```python
from build123d import *

# Parameters (mm, degrees)
SKETCH1_W                  = 812.8
SKETCH1_H                  = 77.724
BOSS_EXTRUDE1_DEPTH        = 22.225
SKETCH2_W                  = 71.374
SKETCH2_H                  = 19.05
CUT_EXTRUDE1_DEPTH         = 817.364663535
HOLE1_D                    = 9.652
HOLE2_D                    = 28.575
H_0_266_DIAMETER_HOLE1_D   = 6.7564
F_10_CLEARANCE_HOLE1_D     = 5.334
F_10_CLEARANCE_HOLE1_DEPTH = 3.175
F_10_CLEARANCE_HOLE2_D     = 5.334
F_10_CLEARANCE_HOLE2_DEPTH = 3.175
F_10_CLEARANCE_HOLE3_D     = 5.334
CHAMFER1_SIZE              = 3.175
FILLET1_R                  = 0.762
FILLET2_R                  = 3.937
CUT_EXTRUDE2_REACH         = 818.445
SKETCH15_W                 = 23.8125
SKETCH15_H                 = 77.724


with BuildPart() as part:
    # Sketch1 → Boss-Extrude1 (new body)
    with BuildSketch(Plane.XZ.offset(19.05)):
        with Locations((406.4, -34.925)):
            Rectangle(SKETCH1_W, SKETCH1_H)
    extrude(amount=-BOSS_EXTRUDE1_DEPTH)

    # Sketch2 → Cut-Extrude1 (cut, through all)
    with BuildSketch(Plane.ZY):
        with Locations((-34.925, -9.525)):
            Rectangle(SKETCH2_W, SKETCH2_H)
    extrude(amount=-CUT_EXTRUDE1_DEPTH, mode=Mode.SUBTRACT)

    # Hole1 (through all)
    with Locations(Plane(origin=(0, 0, 0), x_dir=(-1, 0, 0), z_dir=(0, -1, 0))):
        with Locations((-568.924874752, 19.05), (-601.438495912, 19.05), (-628.947697627, 19.05), (-243.875125248, 19.05), (-211.361504088, 19.05), (-183.852302373, 19.05), (-678.944202666, 20.828), (-701.450372003, 20.828), (-726.460886343, 20.828), (-133.855797334, 20.828), (-111.349627997, 20.828), (-86.339113657, 20.828)):
            Hole(HOLE1_D / 2)

    # Hole2 (through all)
    with Locations(Plane(origin=(0, 0, 0), x_dir=(-1, 0, 0), z_dir=(0, -1, 0))):
        with Locations((-664.970837168, 36.83), (-147.829162832, 36.83), (-406.4, 17.272)):
            Hole(HOLE2_D / 2)

    # H (0.266) Diameter Hole1 (through all)
    with Locations(Plane(origin=(0, 0, 0), x_dir=(-1, 0, 0), z_dir=(0, -1, 0))):
        with Locations((-762, 11.43), (-762, 62.23), (-711.2, 11.43), (-711.2, 62.23), (-660.4, 11.43), (-660.4, 62.23), (-609.6, 11.43), (-609.6, 62.23), (-558.8, 11.43), (-558.8, 62.23), (-152.4, 11.43), (-203.2, 62.23), (-203.2, 11.43), (-254, 62.23), (-50.8, 11.43), (-101.6, 62.23), (-101.6, 11.43), (-152.4, 62.23), (-254, 11.43), (-304.8, 62.23), (-355.6, 62.23), (-355.6, 11.43), (-508, 62.23), (-457.2, 11.43), (-457.2, 62.23), (-406.4, 62.23), (-50.8, 62.23), (-583.538437168, 62.23), (-583.538437168, 11.43), (-229.261562832, 11.43), (-229.261562832, 62.23), (-513.925467617, 17.547282407), (-298.874532383, 17.547282407)):
            Hole(H_0_266_DIAMETER_HOLE1_D / 2)

    # #10 Clearance Hole1
    with Locations(Plane(origin=(0, 0, 0.762), x_dir=(-1, 0, 0), z_dir=(0, 0, -1))):
        with Locations((-12.7, -12.7), (-800.1, -12.7)):
            Hole(F_10_CLEARANCE_HOLE1_D / 2, depth=F_10_CLEARANCE_HOLE1_DEPTH)

    # #10 Clearance Hole2
    with Locations(Plane.XY.offset(3.937)):
        with Locations((63.5, -12.7), (38.1, -12.7), (88.9, -12.7), (114.3, -12.7), (139.7, -12.7), (165.1, -12.7), (190.5, -12.7), (215.9, -12.7), (241.3, -12.7), (266.7, -12.7), (292.1, -12.7), (317.5, -12.7), (342.9, -12.7), (368.3, -12.7), (393.7, -12.7), (419.1, -12.7), (444.5, -12.7), (469.9, -12.7), (495.3, -12.7), (520.7, -12.7), (546.1, -12.7), (571.5, -12.7), (596.9, -12.7), (622.3, -12.7), (647.7, -12.7), (673.1, -12.7), (698.5, -12.7), (723.9, -12.7), (749.3, -12.7), (774.7, -12.7)):
            Hole(F_10_CLEARANCE_HOLE2_D / 2, depth=F_10_CLEARANCE_HOLE2_DEPTH)

    # #10 Clearance Hole3 (through all)
    with Locations(Plane.XY.offset(-70.612)):
        with Locations((800.1, -12.7), (774.7, -12.7), (749.3, -12.7), (723.9, -12.7), (698.5, -12.7), (673.1, -12.7), (647.7, -12.7), (622.3, -12.7), (596.9, -12.7), (571.5, -12.7), (546.1, -12.7), (520.7, -12.7), (495.3, -12.7), (469.9, -12.7), (444.5, -12.7), (419.1, -12.7), (393.7, -12.7), (368.3, -12.7), (342.9, -12.7), (317.5, -12.7), (292.1, -12.7), (266.7, -12.7), (241.3, -12.7), (215.9, -12.7), (190.5, -12.7), (165.1, -12.7), (139.7, -12.7), (114.3, -12.7), (88.9, -12.7), (63.5, -12.7), (38.1, -12.7), (12.7, -12.7)):
            Hole(F_10_CLEARANCE_HOLE3_D / 2)

    # Chamfer1
    chamfer1_edges = [part.edges().sort_by_distance(p)[0] for p in [
        (812.8, -19.05, 2.3495),
        (0, -19.05, -72.1995),
        (0, -19.05, 2.3495),
        (812.8, -19.05, -72.1995),
    ]]
    chamfer(chamfer1_edges, length=CHAMFER1_SIZE)

    # Fillet1
    fillet1_edges = [part.edges().sort_by_distance(p)[0] for p in [
        (406.4, 0, -70.612),
        (406.4, 0, 0.762),
    ]]
    fillet(fillet1_edges, radius=FILLET1_R)

    # Fillet2
    fillet2_edges = [part.edges().sort_by_distance(p)[0] for p in [
        (406.4, 3.175, -73.787),
        (406.4, 3.175, 3.937),
    ]]
    fillet(fillet2_edges, radius=FILLET2_R)

    # Sketch15 → Cut-Extrude2 (cut, up to next)
    with BuildSketch(Plane(origin=(0, 3.175, 0), x_dir=(1, 0, 0), z_dir=(0, 1, 0)), mode=Mode.PRIVATE) as cut_extrude2_sk1:
        with Locations((11.90625, 34.925)):
            Rectangle(SKETCH15_W, SKETCH15_H)
    cut_extrude2_tool1 = extrude(cut_extrude2_sk1.sketch, amount=-CUT_EXTRUDE2_REACH, mode=Mode.PRIVATE) & part.part
    # Sketch15 → Cut-Extrude2 (cut, up to next)
    with BuildSketch(Plane(origin=(0, 3.175, 0), x_dir=(1, 0, 0), z_dir=(0, 1, 0)), mode=Mode.PRIVATE) as cut_extrude2_sk2:
        with Locations((800.89375, 34.925)):
            Rectangle(SKETCH15_W, SKETCH15_H)
    cut_extrude2_tool2 = extrude(cut_extrude2_sk2.sketch, amount=-CUT_EXTRUDE2_REACH, mode=Mode.PRIVATE) & part.part
    add(cut_extrude2_tool1.solids().sort_by_distance((11.90625, 3.175, -34.925))[0], mode=Mode.SUBTRACT)
    add(cut_extrude2_tool2.solids().sort_by_distance((800.89375, 3.175, -34.925))[0], mode=Mode.SUBTRACT)


solid = part.part
```
Part model, mm, in its own coordinate system. A direction names the side the tool comes from. Round coordinates to 2 decimals unless told otherwise and drop trailing zeros.
Item 1: Two-plate mould, pull along Z, no slides. Class faces 3 (the flat face through (401, -10, 0.762)), 4 (the flat face through (401, 0, -35)), 5 (the flat face through (401, -10, -73.787)), 6 (the flat face through (23.812, 0.3, -34.7)): +Z half, -Z half, draft (parallel to the pull), parting line (faces both ways), or undercut.
Results:
face 3: undercut
face 4: undercut
face 5: -Z half
face 6: draft
Item 2: Probe L1, parallel to Z at x = 98.5, y = -5.25; L2, parallel to Z at x = 152.4, y = 0.7; L3, parallel to Y at x = 224, z = -1.5 (3 decimals). List the from-to ranges inside material, lowest first.
Results:
L1: z = -73.79 to -70.61, 0.76 to 3.94
L2: z = -73.51 to -65.61, -58.85 to -50.37, -23.29 to -14.81, -8.05 to 3.66
L3: y = 0 to 3.175
Item 3: Drop a flat-ended pin along its axis: pin 1 Ø4 at (x, z) = (698, -48.5) entering from -Y. Give the stop position or say it passes through.
Results:
pin 1: stops at y = 0
Item 4: Which spindle directions (+Z, -Z, +X, -X, +Y, -Y) get a long thin tool onto all of the face, cutting with end or side? Do faces 1 (the flat face through (401, -10, 3.937)), 2 (the flat face through (401, -10, -70.612)). Say none if no direction does.
Results:
face 1: +Z, +X, -X, +Y, -Y
face 2: +X, -X, -Y
